```python
from build123d import *

# Parameters (mm, degrees)
BOSS_EXTRUDE1_DEPTH = 10
SKETCH3_W           = 5.5
SKETCH3_H           = 10
CUT_EXTRUDE1_DEPTH  = 2.5
CUT_EXTRUDE2_DEPTH  = 28.83597813
CUT_EXTRUDE3_DEPTH  = 2.5
CHAMFER1_SIZE       = 0.4


with BuildPart() as part:
    # Sketch1 → Boss-Extrude1 (new body)
    with BuildSketch(Plane(origin=(0, 0, 0), x_dir=(1, 0, 0), z_dir=(0, 1, 0))):
        with BuildLine():
            Line((15.1, -8.717989065), (15.1, 8.717989065))
            Line((15.1, 8.717989065), (0, 17.43597813))
            Line((0, 17.43597813), (-15.1, 8.717989065))
            Line((-15.1, 8.717989065), (-15.1, 7.2))
            ThreePointArc((-15.1, 7.2), (-16.0372583, 4.9372583), (-18.3, 4))
            Line((-18.3, 4), (-33.4, 4))
            ThreePointArc((-33.4, 4), (-35, 5.6), (-33.4, 7.2))
            Line((-33.4, 7.2), (-27.9, 7.2))
            ThreePointArc((-27.9, 7.2), (-26.132233047, 7.932233047), (-25.4, 9.7))
            Line((-25.4, 9.7), (-18.3, 9.7))
            ThreePointArc((-18.3, 9.7), (-18.176160108, 9.73872205), (-18.096437184, 9.841093781))
            ThreePointArc((-18.096437184, 9.841093781), (-17.541501628, 10.786580324), (-16.7, 11.489270357))
            Line((-16.7, 11.489270357), (-1.6, 20.207259422))
            ThreePointArc((-1.6, 20.207259422), (0, 20.63597813), (1.6, 20.207259422))
            Line((1.6, 20.207259422), (16.7, 11.489270357))
            ThreePointArc((16.7, 11.489270357), (17.871281292, 10.317989065), (18.3, 8.717989065))
            Line((18.3, 8.717989065), (18.3, -8.717989065))
            ThreePointArc((18.3, -8.717989065), (17.871281292, -10.317989065), (16.7, -11.489270357))
            Line((16.7, -11.489270357), (1.6, -20.207259422))
            ThreePointArc((1.6, -20.207259422), (0, -20.63597813), (-1.6, -20.207259422))
            Line((-1.6, -20.207259422), (-16.7, -11.489270357))
            ThreePointArc((-16.7, -11.489270357), (-17.541501628, -10.786580324), (-18.096437184, -9.841093781))
            ThreePointArc((-18.096437184, -9.841093781), (-18.176160108, -9.73872205), (-18.3, -9.7))
            Line((-18.3, -9.7), (-25.4, -9.7))
            ThreePointArc((-25.4, -9.7), (-26.132233047, -7.932233047), (-27.9, -7.2))
            Line((-27.9, -7.2), (-33.4, -7.2))
            ThreePointArc((-33.4, -7.2), (-35, -5.6), (-33.4, -4))
            Line((-33.4, -4), (-18.3, -4))
            ThreePointArc((-18.3, -4), (-16.0372583, -4.9372583), (-15.1, -7.2))
            Line((-15.1, -7.2), (-15.1, -8.717989065))
            Line((-15.1, -8.717989065), (0, -17.43597813))
            Line((0, -17.43597813), (15.1, -8.717989065))
        make_face()
    extrude(amount=BOSS_EXTRUDE1_DEPTH)

    # Sketch3 → Cut-Extrude1 (cut)
    with BuildSketch(Plane(origin=(0, 0, -9.7), x_dir=(-1, 0, 0), z_dir=(0, 0, -1))):
        with Locations((21.05, 5)):
            Rectangle(SKETCH3_W, SKETCH3_H)
    extrude(amount=-CUT_EXTRUDE1_DEPTH, mode=Mode.SUBTRACT)

    # Sketch4 → Cut-Extrude2 (cut, through all)
    with BuildSketch(Plane(origin=(0, 0, -7.2), x_dir=(-1, 0, 0), z_dir=(0, 0, -1))):
        with BuildLine():
            Line((20.25, 6.385640646), (21.05, 6.847520861))
            Line((21.05, 6.847520861), (21.85, 6.385640646))
            ThreePointArc((21.85, 6.385640646), (22.65, 5), (21.85, 3.614359354))
            Line((21.85, 3.614359354), (21.05, 3.152479139))
            Line((21.05, 3.152479139), (20.25, 3.614359354))
            ThreePointArc((20.25, 3.614359354), (19.45, 5), (20.25, 6.385640646))
        make_face()
    extrude(amount=-CUT_EXTRUDE2_DEPTH, mode=Mode.SUBTRACT)

    # Sketch5 → Cut-Extrude3 (cut)
    with BuildSketch(Plane.XY.offset(9.7)):
        with BuildLine():
            Line((-22.425, 2.61843014), (-21.05, 1.824573519))
            Line((-21.05, 1.824573519), (-19.675, 2.61843014))
            ThreePointArc((-19.675, 2.61843014), (-18.3, 5), (-19.675, 7.38156986))
            Line((-19.675, 7.38156986), (-21.05, 8.175426481))
            Line((-21.05, 8.175426481), (-22.425, 7.38156986))
            ThreePointArc((-22.425, 7.38156986), (-23.8, 5), (-22.425, 2.61843014))
        make_face()
    extrude(amount=-CUT_EXTRUDE3_DEPTH, mode=Mode.SUBTRACT)

    # Chamfer1
    chamfer1_edges = [part.edges().sort_by_distance(p)[0] for p in [
        (-30.65, 10, -7.2),
        (-35, 10, -5.6),
        (-25.85, 10, -4),
        (-16.0372583, 10, -4.9372583),
        (-15.1, 10, -7.958994532),
        (-7.55, 10, -13.076983597),
        (7.55, 10, -13.076983597),
        (15.1, 10, 0),
        (-15.1, 10, 7.958994532),
        (-16.0372583, 10, 4.9372583),
        (-25.85, 10, 4),
        (-35, 10, 5.6),
        (-30.65, 10, 7.2),
        (15.1, 0, 0),
        (7.55, 0, -13.076983597),
        (-7.55, 0, -13.076983597),
        (-15.1, 0, -7.958994532),
        (-16.0372583, 0, -4.9372583),
        (-25.85, 0, -4),
        (-35, 0, -5.6),
        (-26.132233047, 10, 7.932233047),
        (-30.65, 0, -7.2),
        (-26.132233047, 0, -7.932233047),
        (-18.176160108, 0, -9.73872205),
        (-17.541501628, 0, -10.786580324),
        (-9.15, 0, -15.848264889),
        (0, 0, -20.63597813),
        (9.15, 0, -15.848264889),
        (17.871281292, 0, -10.317989065),
        (18.3, 0, 0),
        (-21.85, 10, 9.7),
        (17.871281292, 0, 10.317989065),
        (9.15, 0, 15.848264889),
        (0, 0, 20.63597813),
        (-9.15, 0, 15.848264889),
        (-17.541501628, 0, 10.786580324),
        (-18.176160108, 0, 9.73872205),
        (-21.85, 0, 9.7),
        (-26.132233047, 0, 7.932233047),
        (-30.65, 0, 7.2),
        (-35, 0, 5.6),
        (-18.176160108, 10, 9.73872205),
        (-25.85, 0, 4),
        (-16.0372583, 0, 4.9372583),
        (-15.1, 0, 7.958994532),
        (-7.55, 0, 13.076983597),
        (7.55, 0, 13.076983597),
        (-17.541501628, 10, 10.786580324),
        (-9.15, 10, 15.848264889),
        (7.55, 10, 13.076983597),
        (0, 10, 20.63597813),
        (9.15, 10, 15.848264889),
        (17.871281292, 10, 10.317989065),
        (18.3, 10, 0),
        (17.871281292, 10, -10.317989065),
        (9.15, 10, -15.848264889),
        (0, 10, -20.63597813),
        (-9.15, 10, -15.848264889),
        (-17.541501628, 10, -10.786580324),
        (-18.176160108, 10, -9.73872205),
        (-7.55, 10, 13.076983597),
        (-24.6, 0, -9.7),
        (-24.6, 10, -9.7),
        (-18.3, 0, -8.45),
        (-21.05, 10, -7.2),
        (-18.3, 10, -8.45),
        (-23.8, 10, -8.45),
        (-21.05, 0, -7.2),
        (-23.8, 0, -8.45),
        (-26.132233047, 10, -7.932233047),
    ]]
    chamfer(chamfer1_edges, length=CHAMFER1_SIZE)


solid = part.part
```
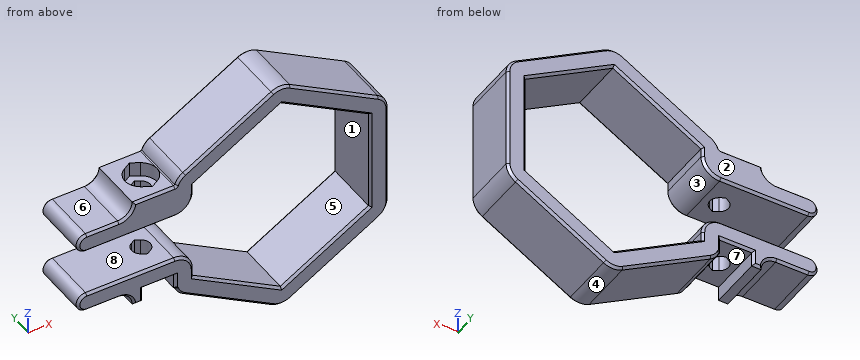
Geometry: final body of the model. Coordinates: model frame, mm. Face numbers are marked on the shaded views. A direction names the side the tool comes from. Give positions to 0.01 mm unless a question says otherwise; leave off trailing zeros. Order: outer loops, then holes, each group sorted by start corner. A loop starts at its lowest first (then second) coordinate and runs counter-clockwise, first axis right, second up. Notation, with made-up numbers: (-28, 75) -> (-20, 75) arc R17 ccw to (-20, 95) -> close; hole circle Ø5 at (65.5, 55). An arc over 180 degrees is marked (long way). Write each question's results on one line, items separated by ' | '. Start each with the question number.
1) Section B-B (z = -13). Return loops of the section in (x, y).
2) Set-up query: the marked faces 5, 6, 7 and 8. Return all of +Z, -Z, +X, -X, +Y, -Y with unobstructed straight access to the full face (end or side cutting, diameter ignored); none if empty.
3) Draft query along Z for the marked faces 1, 2, 3 and 4. Return one class per face: pulls with the +Z half, pulls with the -Z half, needs draft (parallel to the pull), parting line crosses it, or undercut.
4) Section A-A (x = -14). Return loops of the section in (y, z), then the cut area to 3 significant figures.
5) First-contact query: pin 1 (3 mm diameter, centred on x = -28, y = 3, fed in from +Z); pin 2 (4.5 mm diameter, centred on x = -28, y = 7, fed in from -Z); pin 3 (0.8 mm diameter, centred on x = -24.5, y = 2.5, fed in from -Z). Flat tips, straight axial feed; report the tip coordinate or a pass-through.
6) Section C-C (z = 8). Count the separate pieces of the cut face and the enclosed holes in it, then the cut area to 3 significant figures.
7) Line query: line 1 (Z direction, x = -21.5, y = 2.5); line 2 (Z direction, x = -19, y = 8); line 3 (X direction, y = 3.5, z = 10.5). Output: solid intervals per line, ascending. Write a range as from..to.
Calculated:
1) outline: (-14.08, 0.4) -> (-13.28, 0) -> (-8.48, 0) -> (-7.68, 0.4) -> (-7.68, 9.6) -> (-8.48, 10) -> (-13.28, 10) -> (-14.08, 9.6) -> close; (7.68, 0.4) -> (8.48, 0) -> (13.28, 0) -> (14.08, 0.4) -> (14.08, 9.6) -> (13.28, 10) -> (8.48, 10) -> (7.68, 9.6) -> close
2) face 5: +Y, -Y | face 6: +Z, -X, +Y, -Y | face 7: -Z, +Y, -Y | face 8: -X, +Y, -Y
3) face 1: undercut | face 2: needs draft | face 3: undercut | face 4: pulls with the -Z half
4) outline: (0, -12.59) -> (0.4, -13.05) -> (9.6, -13.05) -> (10, -12.59) -> (10, -9.81) -> (9.6, -9.35) -> (0.4, -9.35) -> (0, -9.81) -> close; (0, 9.81) -> (0.4, 9.35) -> (9.6, 9.35) -> (10, 9.81) -> (10, 12.59) -> (9.6, 13.05) -> (0.4, 13.05) -> (0, 12.59) -> close | area: 73.2 mm2
5) pin 1: z = 7.63 | pin 2: z = -8.42 | pin 3: z = -9.7
6) separate pieces: 2 | enclosed holes: 1 | area: 116 mm2
7) line 1: -7.2..-4, 4..7.2 | line 2: -7.2..-4, 4..9.7 | line 3: -17.76..-12.01, 12.01..17.76
